```python
from build123d import *

# Parameters (mm, degrees)
F0_W        = 4.76
F0_H        = 15.24
F0_W_2      = 15.24
F0_R        = 1.95
F1_DEPTH    = 3
F2_DEPTH    = 3
F3_W        = 15.24
F3_H        = 22
F3_R        = 2.2
F3_H_2      = 3
F4_DEPTH    = 3
F5_T1_DEPTH = 38.1528784748
F6_R        = 1


# Not quite as in the source:
# - a fillet or chamfer that OpenCascade refuses, or shapes differently, is made with other operations: its cross-section is extruded or revolved along the edge and cut away or added
# - a feature names something its author has since deleted; it is built from what else it names


with BuildPart() as f1:
    # F0 (on Top) → F1 (new body)
    with BuildSketch(Plane.XY):
        with Locations((-7.62, 0)):
            Rectangle(F0_W, F0_H)
        with Locations((2.38, 0)):
            Rectangle(F0_W_2, F0_H)
        with Locations((2.38, 0)):
            Circle(F0_R, mode=Mode.SUBTRACT)
        with Locations((2.38, 0)):
            Circle(F0_R)
    extrude(amount=F1_DEPTH)

    # F0 (on Top) → F2 (join)
    with BuildSketch(Plane.XY):
        with Locations((2.38, 0)):
            Circle(F0_R)
    extrude(amount=-F2_DEPTH)

    # F3 (on face) → F4 (join)
    with BuildSketch(Plane(origin=(-10, 0, 0), x_dir=(0, -1, 0), z_dir=(-1, 0, 0))):
        with Locations((0, -11)):
            Rectangle(F3_W, F3_H)
        with Locations((0, -18.2633977383)):
            Circle(F3_R, mode=Mode.SUBTRACT)
        with Locations((0, 1.5)):
            Rectangle(F3_W, F3_H_2)
    extrude(amount=F4_DEPTH)

    # F5: fillet of radius 5 on 1 edges, made by hand

    # F5_s2 → F5_t1 (cut)
    with BuildSketch(Plane.XZ.offset(-19.0764392374)):
        with BuildLine():
            ThreePointArc((5.417424305, 0), (8.1560370926, 0.8166998673), (10, 3))
            Line((10, 3), (10, 0))
            Line((10, 0), (5.417424305, 0))
        make_face()
    extrude(amount=F5_T1_DEPTH, mode=Mode.SUBTRACT)

    # F6
    f6_edges = [f1.edges().sort_by_distance(p)[0] for p in [
        (10, 0, 3),
    ]]
    fillet(f6_edges, radius=F6_R)


solid = f1.part
```
Check sheet for the modelled part. Datum: model origin and axes. Units: mm. A direction names the side the tool comes from. Coordinates: 2 decimals unless noted, no trailing zeros. Loops run counter-clockwise (first coordinate to the right, second up) from the corner with the lowest first, then second, coordinate; pieces in that order, holes last.
1) Access from +Z, -Z, +X, -X, +Y, -Y to the whole of each face (thin tool, end or side, straight path). Record for faces 1 (the face through (4.2, -0.7, -1.5)), 2 (the face through (-11.48, 0.48, -20.41)).
2) Sectioned sample at B-B (y = 0). Record the boundary of the cut face in (x, z), and give its area (3 significant figures).
3) Sectioned sample at C-C (x = 2.38). Record the boundary of the cut face in (y, z).
4) Gauge pin test, flat ends, axial feed: pin 1 (5 mm diameter, centred on y = 3, z = -14, fed in from +X); pin 2 (2 mm diameter, centred on x = 2.5, y = -0.5, fed in from -Z); pin 3 (1.5 mm diameter, centred on x = 0, y = -3.5, fed in from -Z). Record the tip position at first contact, or that the pin passes through.
5) Release check for a two-part mould opening along X. For faces 3 (the face through (-13, 0, -9)), 4 (the face through (2, 0, -3)), 5 (the face through (-2, 0, 0)) record: released by +X, released by -X, zero draft, split by the parting line, or undercut.
6) Material ranges on probe 1 along Z at (x, y) = (-11.05, 0); probe 2 along X at (y, z) = (-0.5, -9.25); probe 3 along Z at (x, y) = (-3, -4.75), recorded low to high.
7) Sectioned sample at D-D (y = 4.5). Record the boundary of the cut face in (x, z), and give its area (3 significant figures).
8) Sectioned sample at A-A (z = -0.75). Record the boundary of the cut face in (x, y).
Check sheet entries:
1. face 1: -Z
1. face 2: +X, -X
2. outline: (-13, -22) - (-10, -22) - (-10, -20.46) - (-13, -20.46) - close; (-13, -16.06) - (-10, -16.06) - (-10, 0) - (0.43, 0) - (0.43, -3) - (4.33, -3) - (4.33, 0) - (5.42, 0) arc R5 ccw to (8.72, 1.25) arc R1 ccw to (8.06, 3) - (-13, 3) - close
2. area: 129 mm2
3. outline: (-7.62, 0) - (-1.95, 0) - (-1.95, -3) - (1.95, -3) - (1.95, 0) - (7.62, 0) - (7.62, 3) - (-7.62, 3) - close
4. pin 1: stops at x = -10
4. pin 2: stops at z = -3
4. pin 3: stops at z = 0
5. face 3: released by -X
5. face 4: zero draft
5. face 5: undercut
6. probe 1: z = -22 to -20.46, -16.06 to 3
6. probe 2: x = -13 to -10
6. probe 3: z = 0 to 3
7. outline: (-13, -22) - (-10, -22) - (-10, 0) - (5.42, 0) arc R5 ccw to (8.72, 1.25) arc R1 ccw to (8.06, 3) - (-13, 3) - close
7. area: 130 mm2
8. outline: (-13, -7.62) - (-10, -7.62) - (-10, 7.62) - (-13, 7.62) - close; circle Ø3.9 at (2.38, 0)
